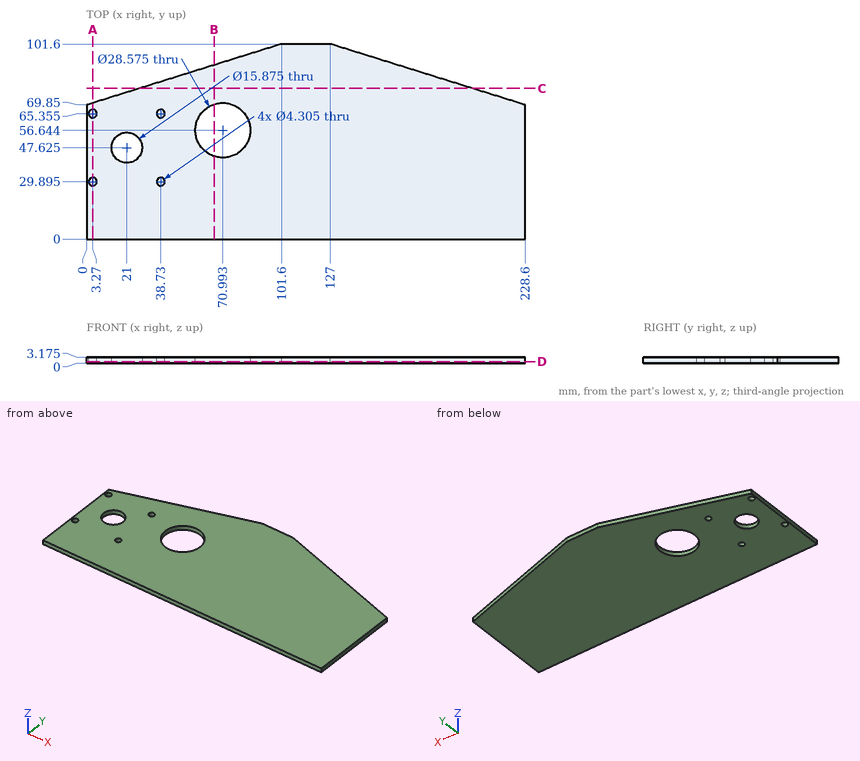
Here's the drawing with two shaded views (mm, measured from the low corner). I have some questions. Coordinates: 2 decimals unless noted, no trailing zeros. Loops run counter-clockwise (first coordinate to the right, second up) from the corner with the lowest first, then second, coordinate; pieces in that order, holes last. Notation, with made-up numbers: (64.5, 85.5) -> (112.5, 85.5) arc R20 cw to (112.5, 124.5) -> close; hole circle Ø2 at (43.25, -12). An arc over 180 degrees is marked (long way). Answer as a JSON object with one key per item and string values.
1) Imagine slicing it at D-D (z = 0.85). Count the separate pieces of the cut face and the enclosed holes in it, then the cut area to 3 significant figures.
Results:
{"separate pieces": "1", "enclosed holes": "6", "area": "19,100 mm^2"}
2) Imagine slicing it at A-A (x = 3.27). Please give me the cut outline in (y, z) (1 decimal), then the cut area to 3 significant figures.
Results:
{"outline": "(0, 0) -> (27.7, 0) -> (27.7, 3.2) -> (0, 3.2) -> close; (32, 0) -> (63.2, 0) -> (63.2, 3.2) -> (32, 3.2) -> close; (67.5, 0) -> (70.9, 0) -> (70.9, 3.2) -> (67.5, 3.2) -> close", "area": "198 mm^2"}
3) Imagine slicing it at C-C (y = 78.5). Please give me the cut outline in (x, z) (1 decimal), then the cut area to 3 significant figures.
Results:
{"outline": "(27.7, 0) -> (200.9, 0) -> (200.9, 3.2) -> (27.7, 3.2) -> close", "area": "550 mm^2"}
4) Imagine slicing it at B-B (x = 66.5). Please give me the cut outline in (y, z) (1 decimal), then the cut area to 3 significant figures.
Results:
{"outline": "(0, 0) -> (43.1, 0) -> (43.1, 3.2) -> (0, 3.2) -> close; (70.2, 0) -> (90.6, 0) -> (90.6, 3.2) -> (70.2, 3.2) -> close", "area": "202 mm^2"}
5) If I drill on line 1 (X direction, y = 57.5, z = 2.2) (1 decimal); line 2 (Y direction, x = 38.73, z = 2.45); line 3 (X direction, y = 59, z = 3.05) (1 decimal), over which ranges is the centre line in solid material (lowest first)?
Results:
{"line 1": "x = 0 to 56.7, 85.3 to 228.6", "line 2": "y = 0 to 27.74, 32.05 to 63.2, 67.51 to 81.95", "line 3": "x = 0 to 56.9, 85.1 to 228.6"}
